CAD build for the part. Positions are in the model's coordinates, mm. Face numbers are marked on the shaded views. A direction names the side the tool comes from. Give positions to 0.01 mm unless a question says otherwise; leave off trailing zeros. Order: outer loops, then holes, each group sorted by start corner. A loop starts at its lowest first (then second) coordinate and runs counter-clockwise, first axis right, second up. Notation, with made-up numbers: M 83.5,71.5 L 113.5,71.5 A35 cw 113.5,104.5 Z; hole C 24.5,-33.5 d4. An arc over 180 degrees is marked long. Put each result on its own line as item: value. Start each with the question number.
1) Pin check, flat tips, straight feed: pin 1 (3 mm diameter, centred on x = -45.5, y = 1.5, fed in from +Z); pin 2 (5 mm diameter, centred on y = 1.5, z = 8, fed in from +X); pin 3 (3 mm diameter, centred on x = -36.5, z = 6.5, fed in from -Y). Stop position of each tip, or through.
2) Two-plate mould, pull along X, no slides. Class the marked faces 4, 5, 6 and 7: released by +X, released by -X, zero draft, split by the parting line, or undercut.
3) Cut at B-B (x = 1). Write the cut outline in (y, z).
4) Tool access for the marked faces 1, 2 and 3: list every direction of +Z, -Z, +X, -X, +Y, -Y with a clear straight run to the whole face (end or side of a thin tool).
5) Drill centre lines: line 1 (X direction, y = 2.5, z = 0.95); line 2 (Y direction, x = -45, z = 0.65); line 3 (X direction, y = -0.5, z = 14). Where is each one in solid material? Low to high. Write a range as [from, to].
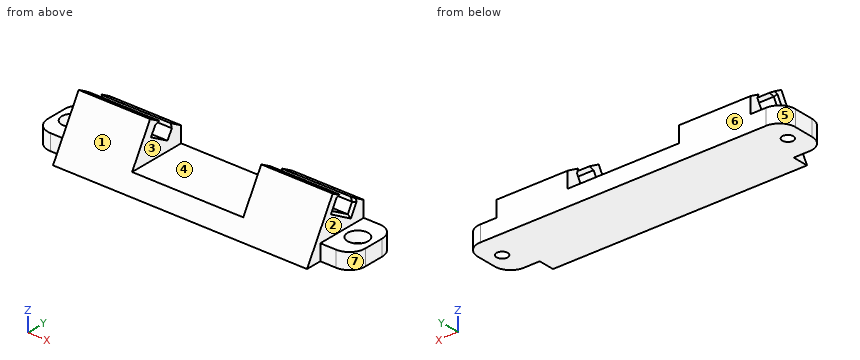
Autodesk Fusion 360 part; units mm, degrees
sketch "Sketch1" plane through (0, 0, 0) normal (1, 0, 0) x (0, 1, 0)
  line L0 (-1.0104, 16.75) -> (-10.681, 0)
  line L1 (-10.681, 0) -> (10.681, 0)
  line L2 (10.681, 0) -> (10.681, 10)
  line L3 (10.681, 10) -> (-1.0104, 16.75)
  line L4 (1.5877, 15.25) -> (-0.5373, 11.5694)
  line L5 (-0.5373, 11.5694) -> (5.5249, 8.0694)
  line L6 (5.5249, 8.0694) -> (7.6499, 11.75)
  line L7 (7.6499, 11.75) -> (1.5877, 15.25) construction
  line L8 (5.5249, 8.0694) -> (-0.5373, 8.0694) construction
  line L9 (-0.5373, 8.0694) -> (-0.5373, 11.5694) construction
  line L10 (10.681, 7.5463) -> (6.5874, 9.9097) construction
  line L11 (0.5252, 13.4097) -> (-2.0729, 14.9097) construction
  line L12 (7.0249, 10.6675) -> (6.5674, 12.375) construction
  line L13 (0.9627, 14.1675) -> (2.6702, 14.625) construction
  dimension "d1" = 30
  dimension "d2" = 7
  dimension "d5" = 10
  dimension "d6" = 3.5
  dimension "d7" = 60
  dimension "d24" = 3
  dimension "d34" = 3
  dimension "d35" = 1.25
  dimension "d36" = 1.25
  dimension "d38" = 45
extrude "Extrude1" add sketch "Sketch1" along normal mid plane 80
sketch "Sketch3" plane through (0, 0, 0) normal (0, 0, 1) x (1, 0, 0)
  line L0 (40, -10.681) -> (40, 10.681)
  line L1 (40, 10.681) -> (45, 10.681)
  line L2 (50, 5.681) -> (50, -0.681)
  line L3 (45, -5.681) -> (40, -5.681)
  line L4 (40, -5.681) -> (40, 10.681)
  arc A0 (50, 5.681) -> (45, 10.681) centre (45, 5.681) ccw
  arc A1 (45, -5.681) -> (50, -0.681) centre (45, -0.681) ccw
  dimension "d11" = 5
  dimension "d12" = 10
  dimension "d15" = 5
extrude "Extrude2" add sketch "Sketch3" along normal blind 5
sketch "Sketch4" plane through (0, 0, 5) normal (0, 0, 1) x (-1, 0, 0)
  line L0 (-40, 5.681) -> (-45, 5.681)
  arc A0 (-45, 5.681) -> (-50, 0.681) centre (-45, 0.681) ccw
  line L1 (-50, 0.681) -> (-50, -5.681)
  arc A1 (-50, -5.681) -> (-45, -10.681) centre (-45, -5.681) ccw
  line L2 (-45, -10.681) -> (-40, -10.681)
  line L3 (-40, -10.681) -> (-40, 5.681)
  circle A2 centre (-45, -2.5) radius 1.75
  line L4 (-45, -10.681) -> (-45, 5.681) construction
  line L5 (-40, -10.681) -> (-50, -10.681) construction
  line L6 (-50, -5.681) -> (-50, -10.681) construction
  dimension "d16" = 3.5
extrude "Extrude3" cut sketch "Sketch4" against normal up to surface (5 mm away) contours A2
chamfer "Chamfer1" distance 1.5 angle 60 1 edges at (46.6316, 1.8672, 5) measured on face at (43.0417, -3.4592, 5)
mirror "Mirror1" about plane through (0, 0, 0) normal (1, 0, 0) of "Extrude2", "Extrude3", "Chamfer1"
sketch "Sketch5" plane through (40, 0, 0) normal (1, 0, 0) x (0, 1, 0)
  line L0 (-5.681, 0) -> (-5.681, 5)
  line L1 (-5.681, 5) -> (10.681, 5)
  line L2 (10.681, 5) -> (10.681, 10)
  line L3 (10.681, 10) -> (-1.0104, 16.75)
  line L4 (-1.0104, 16.75) -> (-10.681, 0)
  line L5 (-10.681, 0) -> (-5.681, 0)
  line L6 (1.5877, 15.25) -> (-0.5373, 11.5694) construction
  line L7 (-0.5373, 11.5694) -> (5.5249, 8.0694) construction
  line L8 (5.5249, 8.0694) -> (7.6499, 11.75) construction
  line L9 (1.5011, 15.3) -> (-0.6739, 11.5328)
  line L10 (-0.6739, 11.5328) -> (5.5615, 7.9328)
  line L11 (5.5615, 7.9328) -> (7.7365, 11.7)
  line L12 (0.9261, 14.3041) -> (2.497, 14.725)
  line L13 (7.1615, 10.7041) -> (6.7406, 12.275)
  dimension "d25" = 0.1
  dimension "d26" = 45
  dimension "d27" = 1.15
  dimension "d28" = 1.15
extrude "Extrude4" cut sketch "Sketch5" against normal up to surface (80 mm away) contours L3 L9 L10 L11 L12 L13
sketch "Sketch6" plane through (0, 0, 0) normal (0, 1, 0) x (1, 0, 0)
  line L0 (-40, -16.75) -> (40, -16.75)
  line L1 (-17.5, -16.75) -> (17.5, -16.75)
  line L2 (17.5, -16.75) -> (17.5, -5)
  line L3 (17.5, -5) -> (-17.5, -5)
  line L4 (-17.5, -5) -> (-17.5, -16.75)
  line L5 (40, -5) -> (45, -5)
  dimension "d32" = 35
extrude "Extrude5" cut sketch "Sketch6" along normal through all and the other way through all
chamfer "Chamfer2" distance 0.75 angle 45 6 edges at (40, 0.1261, 12.9184) (40, 2.4438, 9.7328) (40, 6.3615, 9.3184) (-40, 2.4438, 9.7328) (-40, 0.1261, 12.9184) (-40, 6.3615, 9.3184)
chamfer "Chamfer3" distance 0.75 angle 45 4 edges at (40, 1.1993, 14.3773) (40, 7.0883, 10.9773) (-40, 7.0883, 10.9773) (-40, 1.1993, 14.3773)
Solution:
1. pin 1: z = 3.91
1. pin 2: x = 40
1. pin 3: y = -7.79
2. face 4: undercut
2. face 5: released by -X
2. face 6: zero draft
2. face 7: released by +X
3. outline: M -10.68,0 L 10.68,0 L 10.68,5 L -7.79,5 Z
4. face 1: +Z, +X, -X, -Y
4. face 2: +Z, +X, -Y
4. face 3: +Z, +Y, -Y
5. line 1: [-50, -46.75], [-43.25, 43.25], [46.75, 50]
5. line 2: [-5.68, 0.75], [4.25, 10.68]
5. line 3: [-40, -17.5], [17.5, 40]
